Source: CAD feature listing. Evaluate the final solid. Frame: model axes, mm. Face numbers are marked on the shaded views. A direction names the side the tool comes from. Coordinates: 2 decimals unless noted, no trailing zeros. Write each loop counter-clockwise with the first axis right and the second up, starting at its lowest first coordinate (ties: lowest second). Pieces come first, ordered by that corner, then holes. Notation, with made-up numbers: (-5, 32) - (-1, 32) arc R17 cw to (-1, 42) - close; hole circle Ø1 at (22.5, 87). An arc over 180 degrees is marked (long way). One line per question, with ' | ' between items.
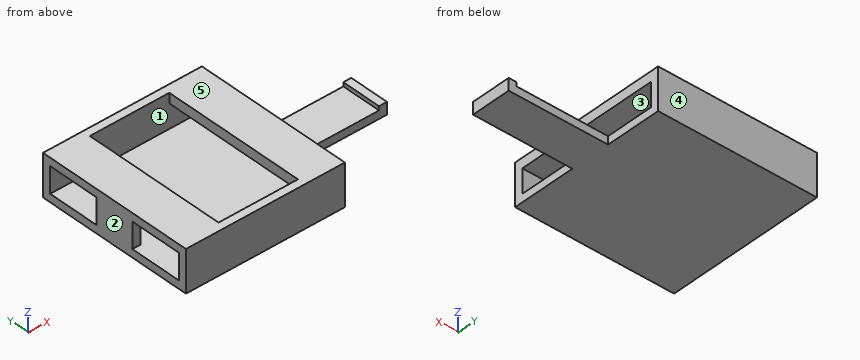
from build123d import *

# Parameters (mm, degrees)
BOX001_W     = 40
BOX001_H     = 36
BOX001_DEPTH = 2
BOX002_W     = 10
BOX002_H     = 38
BOX002_DEPTH = 2.5
BOX003_W     = 40
BOX003_H     = 2
BOX003_DEPTH = 10.5
BOX004_W     = 40
BOX004_H     = 2
BOX004_DEPTH = 10.5
BOX005_W     = 2
BOX005_H     = 10
BOX005_DEPTH = 8.5
BOX006_W     = 63
BOX006_H     = 10
BOX006_DEPTH = 2
BOX007_W     = 2
BOX007_H     = 10
BOX007_DEPTH = 2
BOX_W        = 10
BOX_H        = 38
BOX_DEPTH    = 2


with BuildPart() as cube001:
    # Box001 → Box001 (new body)
    with BuildSketch(Plane(origin=(0, -1, -6), x_dir=(1, 0, 0), z_dir=(0, 0, 1))):
        with Locations((20, 18)):
            Rectangle(BOX001_W, BOX001_H)
    extrude(amount=BOX001_DEPTH)


with BuildPart() as cube002:
    # Box002 → Box002 (new body)
    with BuildSketch(Plane(origin=(30, -2, 2), x_dir=(1, 0, 0), z_dir=(0, 0, 1))):
        with Locations((5, 19)):
            Rectangle(BOX002_W, BOX002_H)
    extrude(amount=BOX002_DEPTH)


with BuildPart() as cube003:
    # Box003 → Box003 (new body)
    with BuildSketch(Plane(origin=(0, -3, -6), x_dir=(1, 0, 0), z_dir=(0, 0, 1))):
        with Locations((20, 1)):
            Rectangle(BOX003_W, BOX003_H)
    extrude(amount=BOX003_DEPTH)


with BuildPart() as cube004:
    # Box004 → Box004 (new body)
    with BuildSketch(Plane(origin=(0, 35, -6), x_dir=(1, 0, 0), z_dir=(0, 0, 1))):
        with Locations((20, 1)):
            Rectangle(BOX004_W, BOX004_H)
    extrude(amount=BOX004_DEPTH)


with BuildPart() as cube005:
    # Box005 → Box005 (new body)
    with BuildSketch(Plane(origin=(0, 12, -4), x_dir=(1, 0, 0), z_dir=(0, 0, 1))):
        with Locations((1, 5)):
            Rectangle(BOX005_W, BOX005_H)
    extrude(amount=BOX005_DEPTH)


with BuildPart() as cube006:
    # Box006 → Box006 (new body)
    with BuildSketch(Plane(origin=(2, 13, -6), x_dir=(1, 0, 0), z_dir=(0, 0, 1))):
        with Locations((31.5, 5)):
            Rectangle(BOX006_W, BOX006_H)
    extrude(amount=BOX006_DEPTH)


with BuildPart() as cube007:
    # Box007 → Box007 (new body)
    with BuildSketch(Plane(origin=(63, 13, -5), x_dir=(1, 0, 0), z_dir=(0, 0, 1))):
        with Locations((1, 5)):
            Rectangle(BOX007_W, BOX007_H)
    extrude(amount=BOX007_DEPTH)


with BuildPart() as fusion:
    # Box → Box (new body)
    with BuildSketch(Plane(origin=(0, -2, 2.5), x_dir=(1, 0, 0), z_dir=(0, 0, 1))):
        with Locations((5, 19)):
            Rectangle(BOX_W, BOX_H)
    extrude(amount=BOX_DEPTH)

    # Fusion: union Cube001, Cube002, Cube003, Cube004, Cube005, Cube006, Cube007
    add(cube001.part)
    add(cube002.part)
    add(cube003.part)
    add(cube004.part)
    add(cube005.part)
    add(cube006.part)
    add(cube007.part)


solid = fusion.part
Item 1: Cut plane B-B on x = 4. Return loops of the section in (y, z).
Check sheet entries:
outline: (-3, -6) - (37, -6) - (37, 4.5) - (-3, 4.5) - close; hole (-1, -4) - (35, -4) - (35, 2.5) - (-1, 2.5) - close
Item 2: Cut plane C-C on z = -1.5. Return loops of the section in (x, y), and give its area (3 significant figures).
Check sheet entries:
outline: (0, -3) - (40, -3) - (40, -1) - (0, -1) - close; (0, 12) - (2, 12) - (2, 22) - (0, 22) - close; (0, 35) - (40, 35) - (40, 37) - (0, 37) - close | area: 180 mm²
Item 3: Cut plane D-D on y = 16.5. Return loops of the section in (x, z), and give its area (3 significant figures).
Check sheet entries:
outline: (0, -6) - (65, -6) - (65, -3) - (63, -3) - (63, -4) - (2, -4) - (2, 2.5) - (10, 2.5) - (10, 4.5) - (0, 4.5) - close; (30, 2) - (40, 2) - (40, 4.5) - (30, 4.5) - close | area: 190 mm²
Item 4: Pin query (flat end, axial travel): pin 1 Ø3.5 at (x, z) = (56.5, -4) entering from +Y; pin 2 Ø1.6 at (x, y) = (64, 18) entering from +Z; pin 3 Ø3.5 at (x, z) = (58.5, -4) entering from -Y; pin 4 Ø6 at (x, z) = (57, 1) entering from +Y. Return the tip coordinate at first contact, or that it passes through.
Check sheet entries:
pin 1: y = 23 | pin 2: z = -3 | pin 3: y = 13 | pin 4: through
Item 5: Access query for the marked faces 1 and 2. Directions: +Z, -Z, +X, -X, +Y, -Y. A direction counts if a zero-diameter tool reaches every point of the face in a straight line with its end or side. Return the directions, or none.
Check sheet entries:
face 1: none | face 2: +Z, -Z, -X, +Y, -Y
Item 6: Mould query, pull axis Y, two halves, no side actions, for the marked faces 3, 4 and 5. Classes: pulls with the +Y half, pulls with the -Y half, needs draft (parallel to the pull), parting line crosses it, or undercut.
Check sheet entries:
face 3: undercut | face 4: pulls with the +Y half | face 5: needs draft
Item 7: Cut plane A-A on y = 32. Return loops of the section in (x, z), and give its area (3 significant figures).
Check sheet entries:
outline: (0, -6) - (40, -6) - (40, -4) - (0, -4) - close; (0, 2.5) - (10, 2.5) - (10, 4.5) - (0, 4.5) - close; (30, 2) - (40, 2) - (40, 4.5) - (30, 4.5) - close | area: 125 mm²
Item 8: Ray query, line 1 along Z through (x, y) = (35, 22); line 2 along Y through (x, z) = (10.5, 1.75); line 3 along X through (y, z) = (20.5, -3.75). Return the intervals inside material, ascending. Write a range as [from, to].
Check sheet entries:
line 1: [-6, -4], [2, 4.5] | line 2: [-3, -1], [35, 37] | line 3: [0, 2], [63, 65]
